from build123d import *

# Parameters (mm, degrees)
F1_DEPTH = 60
F3_DEPTH = 60.001
F5_DEPTH = 80.001


with BuildPart() as f1:
    # F0 (on Top) → F1 (new body)
    with BuildSketch(Plane.XY):
        Polygon((-30, 40), (-30, -40), (30, -40), (30, 40), (22, 40), (22, 36), (22, -30), (-25, -30), (-25, 36), (-25, 40), align=None)
    extrude(amount=F1_DEPTH)

    # F2 (on face) → F3 (cut, through all)
    with BuildSketch(Plane.YZ.offset(30)):
        Polygon((3, 45), (-19.5, 30), (3, 15), (25.5, 30), align=None)
    extrude(amount=-F3_DEPTH, mode=Mode.SUBTRACT)

    # F4 (on face) → F5 (cut, through all)
    with BuildSketch(Plane(origin=(0, 40, 0), x_dir=(-1, 0, 0), z_dir=(0, 1, 0))):
        Polygon((14, 30), (1.5, 50), (-11, 30), (1.5, 10), align=None)
    extrude(amount=-F5_DEPTH, mode=Mode.SUBTRACT)


solid = f1.part
Design review of the part built by this model. Coordinates are the model's own, in mm. A direction names the side the tool comes from. Round coordinates to 2 decimals unless told otherwise and drop trailing zeros. Write each loop counter-clockwise with the first axis right and the second up, starting at its lowest first coordinate (ties: lowest second). Pieces come first, ordered by that corner, then holes. Notation, with made-up numbers: (74, 76) -> (106, 76) arc R32 ccw to (106, 107) -> close; hole circle Ø9 at (89.25, -15.5). An arc over 180 degrees is marked (long way). One line per question, with ' | ' between items.
(1) Take a section at B-B, the plane y = 27.5. State the section outline as (x, z) points, and give its area (3 significant figures).
Result sheet:
outline: (-30, 0) -> (-25, 0) -> (-25, 60) -> (-30, 60) -> close; (22, 0) -> (30, 0) -> (30, 60) -> (22, 60) -> close | area: 780 mm2
(2) Take a section at D-D, the plane z = 52. State the section outline as (x, y) points.
Result sheet:
outline: (-30, -40) -> (30, -40) -> (30, 40) -> (22, 40) -> (22, -30) -> (-25, -30) -> (-25, 40) -> (-30, 40) -> close
(3) Wall thickness on line 1 (X direction, y = -18, z = 23); line 2 (Y direction, x = -8, z = 54.5); line 3 (X direction, y = -31.5, z = 18): over which ranges is each line inside the solid? List them lowest first. Write a range as [from, to].
Result sheet:
line 1: [-30, -25], [22, 30] | line 2: [-40, -30] | line 3: [-30, -6.5], [3.5, 30]
(4) Draft analysis for pull direction Z (two halves, no side actions). For faces 4 (the flat face through (-27.5, -8.4, 22.6)), 5 (the flat face through (24, -12, 60)), 6 (the flat face through (13, -40, 30)), 7 (the flat face through (26.1, -8.4, 22.6)), state which applies: released by +Z, released by -Z, zero draft, split by the parting line, or undercut.
Result sheet:
face 4: undercut | face 5: released by +Z | face 6: zero draft | face 7: undercut
(5) Machinability: for faces 1 (the flat face through (-27.5, -8.1, 37.6)), 2 (the flat face through (-7.663, -34.93, 19.86)), 3 (the flat face through (22, 5, 16)), which of the approach directions +Z, -Z, +X, -X, +Y, -Y give a long, thin tool a straight path to every point of the face, cutting with its end or side? Answer none if there is none.
Result sheet:
face 1: +X, -X | face 2: +Y, -Y | face 3: +Z, -Z, +Y
(6) Insertion check: P1, Ø12, axis at x = -5.5, z = 23, coming from the -Y side; P2, Ø10, axis at x = -7, z = 50.5, coming from the +Y side. Each pin has a flat end and moves straight along its axis. Give the tip position at first contact, or say it passes through.
Result sheet:
P1: y = -40 | P2: y = -30
(7) Take a section at A-A, the plane x = 2. State the section outline as (y, z) points, and give its area (3 significant figures).
Result sheet:
outline: (-40, 0) -> (-30, 0) -> (-30, 15.6) -> (-40, 15.6) -> close; (-40, 44.4) -> (-30, 44.4) -> (-30, 60) -> (-40, 60) -> close | area: 312 mm2
(8) Take a section at C-C, the plane x = 26. State the section outline as (y, z) points.
Result sheet:
outline: (-40, 0) -> (40, 0) -> (40, 60) -> (-40, 60) -> close; hole (-19.5, 30) -> (3, 15) -> (25.5, 30) -> (3, 45) -> close
